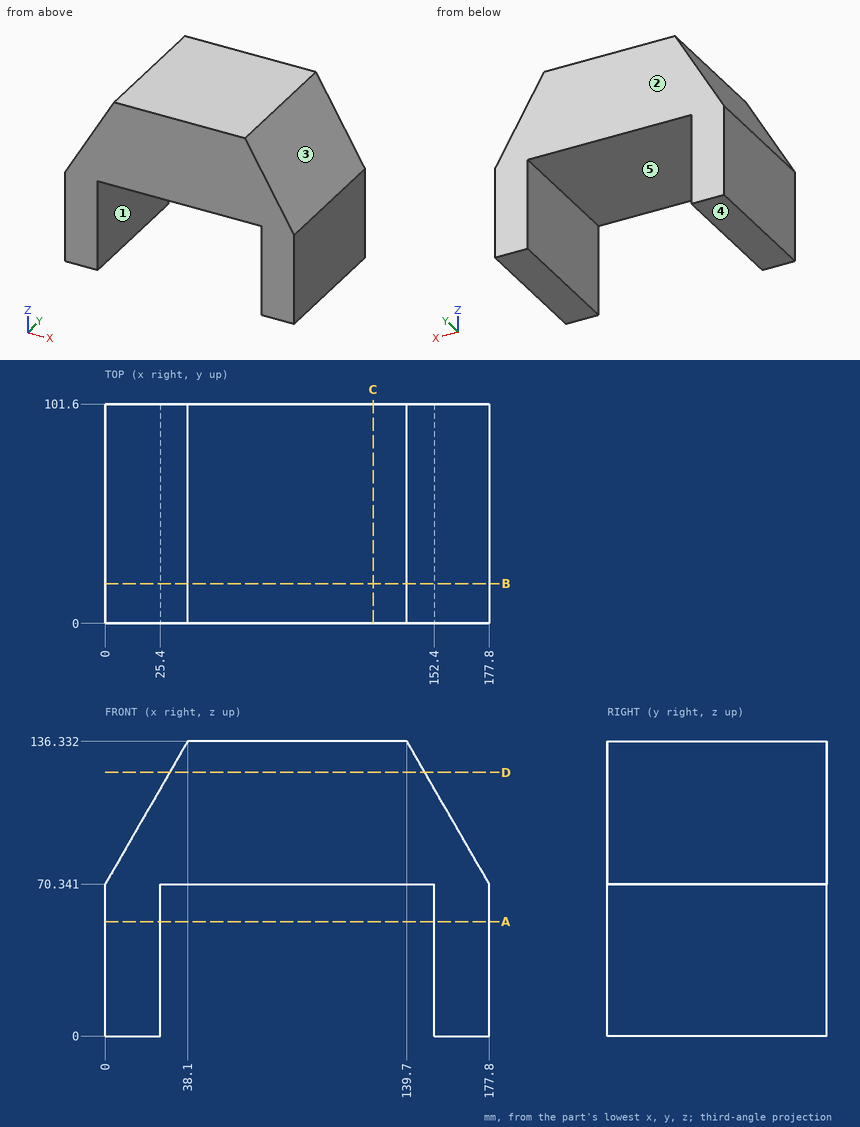
Input: dimensioned drawing with shaded views. Units: mm. Origin: part minimum x, y, z. A direction names the side the tool comes from. Give positions to 0.01 mm unless a question says otherwise; leave off trailing zeros. Write each loop counter-clockwise with the first axis right and the second up, starting at its lowest first coordinate (ties: lowest second). Pieces come first, ordered by that corner, then holes.
Q1. Set-up query: the marked faces 4 and 5. Return all of +Z, -Z, +X, -X, +Y, -Y with unobstructed straight access to the full face (end or side cutting, diameter ignored); none if empty.
Q2. Section D-D, the plane z = 122. Output: boundary loops of the cut face in (x, y) (1 decimal).
Q3. Section B-B, the plane y = 18.5. Output: boundary loops of the cut face in (x, z).
Q4. Pull-direction query (X, two-part tool) for the marked faces 1, 2 and 3; classes: pulls with the +X half, pulls with the -X half, needs draft (parallel to the pull), parting line crosses it, or undercut.
Q5. Material intervals for probe 1 along X at (y, z) = (25.5, 22); probe 2 along Z at (x, y) = (74.5, 17); probe 3 along Z at (x, y) = (155.5, 49) (1 decimal), sorted ascending.
Q6. Section C-C, the plane x = 124. Output: boundary loops of the cut face in (y, z), plus the area to 3 significant figures.
Q7. Section A-A, the plane z = 53. Output: boundary loops of the cut face in (x, y), plus the area to 3 significant figures.
Q8. First-contact query: P1, Ø10, axis at x = 140, y = 18.5, coming from the -Z side; P2, Ø1.5, axis at y = 16, z = 107, coming from the +X side; P3, Ø1, axis at x = 158.5, y = 61.5, coming from the +Z side (1 decimal). Flat tips, straight axial feed; report the tip coordinate or a pass-through.
Filled in:
1. face 4: -Z, +X, -X, +Y, -Y
1. face 5: -Z, +Y, -Y
2. outline: (29.8, 0) - (148, 0) - (148, 101.6) - (29.8, 101.6) - close
3. outline: (0, 0) - (25.4, 0) - (25.4, 70.34) - (152.4, 70.34) - (152.4, 0) - (177.8, 0) - (177.8, 70.34) - (139.7, 136.33) - (38.1, 136.33) - (0, 70.34) - close
4. face 1: undercut
4. face 2: needs draft
4. face 3: pulls with the +X half
5. probe 1: x = 0 to 25.4, 152.4 to 177.8
5. probe 2: z = 70.34 to 136.33
5. probe 3: z = 0 to 109
6. outline: (0, 70.34) - (101.6, 70.34) - (101.6, 136.33) - (0, 136.33) - close
6. area: 6,700 mm2
7. outline: (0, 0) - (25.4, 0) - (25.4, 101.6) - (0, 101.6) - close; (152.4, 0) - (177.8, 0) - (177.8, 101.6) - (152.4, 101.6) - close
7. area: 5,160 mm2
8. P1: stops at z = 70.34
8. P2: stops at x = 157.07
8. P3: stops at z = 104.6
